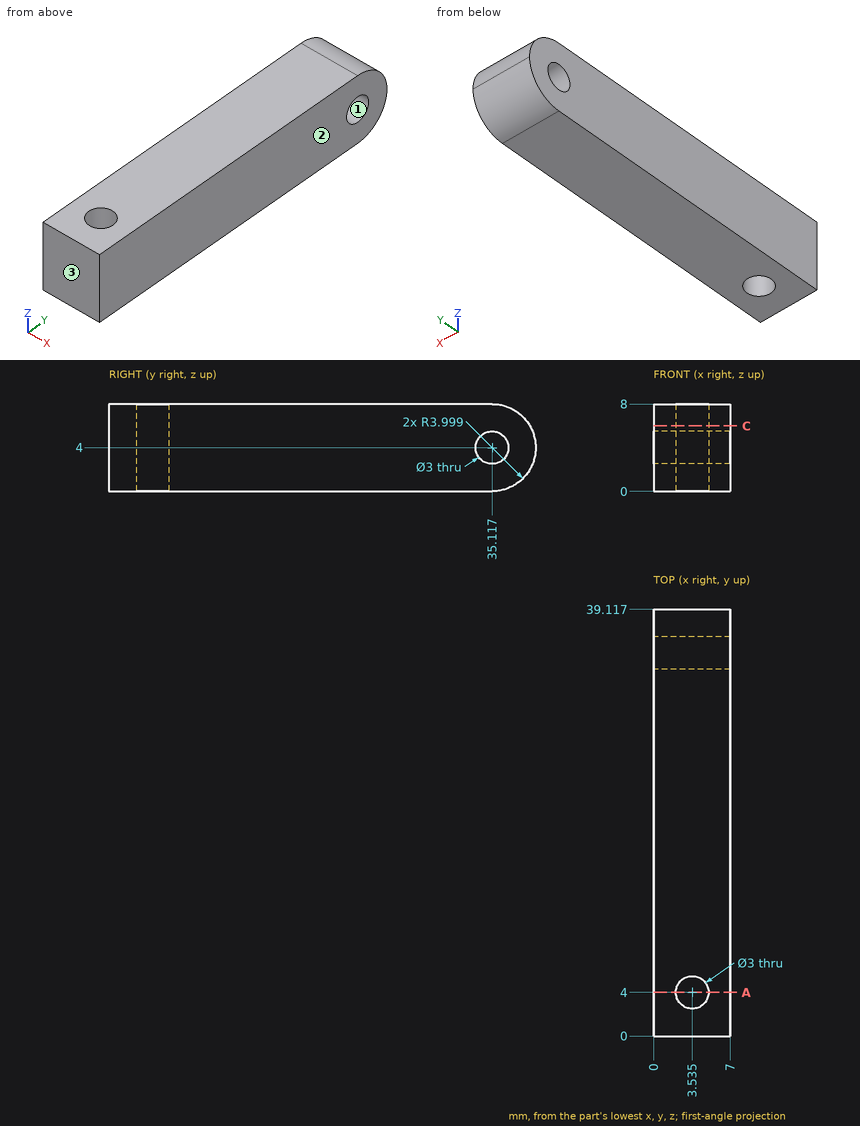
Source: three-view drawing plus pictorial views. Frame: mm from the lowest corner of the part. Coordinates: 2 decimals unless noted, no trailing zeros. Loops run counter-clockwise (first coordinate to the right, second up) from the corner with the lowest first, then second, coordinate; pieces in that order, holes last. Notation, with made-up numbers: (17.25, -37) - (25.25, -37) arc R16 ccw to (25.25, -10) - close; hole circle Ø3 at (70, 63). An arc over 180 degrees is marked (long way). Answer in a Markdown table with one row per item. Add a question column.
Item 1: Line query: line 1 along X through (y, z) = (4, 2.25) (1 decimal); line 2 along Y through (x, z) = (2, 4); line 3 along Y through (x, z) = (2.5, 6.75) (1 decimal). Output: solid intervals per line, ascending. Write a range as [from, to].
Item 2: Section query C-C on z = 6. Return the cut outline in (x, y) (1 decimal).
Item 3: Mould query, pull axis Y, two halves, no side actions, for the marked faces 1, 2 and 3. Classes: released by +Y, released by -Y, zero draft, split by the parting line, or undercut.
Item 4: Contact query for a flat-ended pin moving along its axis: P1, Ø1, axis at x = 5.5, z = 1.5, coming from the +Y side. Output: stop coordinate, or through.
Item 5: Section query A-A on y = 4. Return the cut outline in (x, z) (1 decimal), then the cut area to 3 significant figures.
Recorded:
| question | item | result |
|---|---|---|
| 1 | line 1 | [0, 2], [5, 7] |
| 1 | line 2 | [0, 33.62], [36.62, 39.12] |
| 1 | line 3 | [0, 2.9], [5.1, 38] |
| 2 | outline | (0, 0) - (7, 0) - (7, 38.6) - (0, 38.6) - close; hole circle Ø3 at (3.5, 4) |
| 3 | face 1 | undercut |
| 3 | face 2 | zero draft |
| 3 | face 3 | released by -Y |
| 4 | P1 | y = 38.58 |
| 5 | outline | (0, 0) - (2, 0) - (2, 8) - (0, 8) - close; (5, 0) - (7, 0) - (7, 8) - (5, 8) - close |
| 5 | area | 32.0 mm^2 |
